The model under review builds one solid part; all positions refer to its coordinate system, in mm. A direction names the side the tool comes from. Give positions to 0.01 mm unless a question says otherwise; leave off trailing zeros. Loops run counter-clockwise (first coordinate to the right, second up) from the corner with the lowest first, then second, coordinate; pieces in that order, holes last. Notation, with made-up numbers: M 57,-39.75 L 100,-39.75 A20 ccw 100,-2.75 Z; hole C 65,72.5 d4. An arc over 180 degrees is marked long. One line per item, written item: value. Start each with the question number.
Q1. For faces 4 (the face through (-3, -3, -9.652)), 5 (the face through (0, 0, 38.1)), 6 (the face through (0, -1.524, -23)), list the 3-axis set-ups (+Z, -Z, +X, -X, +Y, -Y) from which the entire face can be reached by the end or side of a thin tool; tool diameter is ignored.
Q2. To check wall thickness, follow line 1 along Z through (x, y) = (0, -2.9); line 2 along Z through (x, y) = (3.5, 5.5); line 3 along X through (y, z) = (-1.5, -11.5). State the ranges of each line that lie inside material, in increasing order. Write a range as from..to.
Q3. We need section A-A on x = 0. Write out the cut boundary in (y, z) (3 decimals), plus the area to 3 significant figures.
Q4. Mouldability with a two-part tool opening along Y and no side actions: class faces 1 (the face through (1.42, -2.73, -24.56)), 2 (the face through (0, 0, -20.066)), 3 (the face through (-6.1, -2.53, -4.76)) as released by +Y, released by -Y, zero draft, split by the parting line, or undercut.
Q5. We need section D-D on z = -22. Write out the cut boundary in (x, y), plus the area to 3 significant figures.
Q6. For pin 1 (1.5 mm diameter, centred on y = 6, z = -9.5, fed in from +X); pin 2 (1.5 mm diameter, centred on x = 0, y = -0.5, fed in from -Z); pin 3 (1.8 mm diameter, centred on x = 0, z = -25.146, fed in from +Y); pin 4 (10 mm diameter, centred on x = -5.5, z = -21, fed in from -Y), all flat-tipped, find the tip position at first contact; note any pin that passes through.
Q7. We need section B-B on y = -3. Write out the cut boundary in (x, z), plus the area to 3 significant figures.
Q8. We need section C-C on y = 0. Write out the cut boundary in (x, z) (3 decimals).
```python
from build123d import *

# Parameters (mm, degrees)
SKETCH1_R               = 9.525
EXTRUDE1_DEPTH          = 38.1
SKETCH2_R               = 6.604
EXTRUDE2_DEPTH          = 9.652
SKETCH3_R               = 3.9751
EXTRUDE3_DEPTH          = 19.05
SKETCH4_W               = 10.16
SKETCH4_H               = 3.048
CUT_EXTRUDE1_DEPTH      = 8.636
SKETCH5_R               = 1.5367
CUT_EXTRUDE2_DEPTH      = 10.525
CUT_EXTRUDE2_DEPTH_BACK = 10.525


with BuildPart() as part:
    # Sketch1 → Extrude1 (new body)
    with BuildSketch(Plane.XY):
        Circle(SKETCH1_R)
    extrude(amount=EXTRUDE1_DEPTH)

    # Sketch2 → Extrude2 (add)
    with BuildSketch(Plane(origin=(0, 0, 0), x_dir=(-1, 0, 0), z_dir=(0, 0, -1))):
        Circle(SKETCH2_R)
    extrude(amount=EXTRUDE2_DEPTH)

    # Sketch3 → Extrude3 (add)
    with BuildSketch(Plane(origin=(0, 0, -9.652), x_dir=(-1, 0, 0), z_dir=(0, 0, -1))):
        Circle(SKETCH3_R)
    extrude(amount=EXTRUDE3_DEPTH)

    # Sketch4 → Cut-Extrude1 (cut)
    with BuildSketch(Plane(origin=(0, 0, -28.702), x_dir=(-1, 0, 0), z_dir=(0, 0, -1))):
        with Locations((0.063992248, 0)):
            Rectangle(SKETCH4_W, SKETCH4_H)
    extrude(amount=-CUT_EXTRUDE1_DEPTH, mode=Mode.SUBTRACT)

    # Sketch5 → Cut-Extrude2 (cut, two sides)
    with BuildSketch(Plane(origin=(0, 0, 0), x_dir=(1, 0, 0), z_dir=(0, 1, 0))) as cut_extrude2_sk:
        with Locations((0, 25.146)):
            Circle(SKETCH5_R)
    extrude(amount=CUT_EXTRUDE2_DEPTH, mode=Mode.SUBTRACT)
    extrude(cut_extrude2_sk.sketch, amount=-CUT_EXTRUDE2_DEPTH_BACK, mode=Mode.SUBTRACT)


solid = part.part
```
Solved:
1. face 4: -Z
1. face 5: +Z, +X, -X, +Y, -Y
1. face 6: -Z, +X, -X
2. line 1: -28.7..-26.68, -23.61..38.1
2. line 2: -9.65..38.1
2. line 3: -3.68..3.68
3. outline: M -9.525,0 L -6.604,0 L -6.604,-9.652 L -3.975,-9.652 L -3.975,-23.609 L -1.524,-23.609 L -1.524,-20.066 L 1.524,-20.066 L 1.524,-23.609 L 3.975,-23.609 L 3.975,-9.652 L 6.604,-9.652 L 6.604,0 L 9.525,0 L 9.525,38.1 L -9.525,38.1 Z; M -3.975,-28.702 L -1.524,-28.702 L -1.524,-26.683 L -3.975,-26.683 Z; M 1.524,-28.702 L 3.975,-28.702 L 3.975,-26.683 L 1.524,-26.683 Z
3. area: 963 mm2
4. face 1: zero draft
4. face 2: undercut
4. face 3: split by the parting line
5. outline: M -3.67,-1.52 A3.98 ccw 3.67,-1.52 Z; M -3.67,1.52 L 3.67,1.52 A3.98 ccw Z
5. area: 26.0 mm2
6. pin 1: x = 4.01
6. pin 2: z = -20.07
6. pin 3: through
6. pin 4: y = -3.94
7. outline: M -9.04,0 L -5.88,0 L -5.88,-9.65 L -2.61,-9.65 L -2.61,-28.7 L 2.61,-28.7 L 2.61,-9.65 L 5.88,-9.65 L 5.88,0 L 9.04,0 L 9.04,38.1 L -9.04,38.1 Z; hole C 0,-25.15 d3.07
7. area: 894 mm2
8. outline: M -9.525,0 L -6.604,0 L -6.604,-9.652 L -3.975,-9.652 L -3.975,-20.066 L 3.975,-20.066 L 3.975,-9.652 L 6.604,-9.652 L 6.604,0 L 9.525,0 L 9.525,38.1 L -9.525,38.1 Z
